```python
from build123d import *

# Parameters (mm, degrees)
BOSS_EXTRUDE1_DEPTH      = 1.5
BOSS_EXTRUDE1_DEPTH_BACK = 1.5
BOSS_EXTRUDE2_DEPTH      = 1.5
BOSS_EXTRUDE2_DEPTH_BACK = 1.5
SKETCH4_W                = 11.052180397
SKETCH4_H                = 1.65
SKETCH5_R                = 1.4
BOSS_EXTRUDE20_DEPTH     = 3.5
SKETCH6_R                = 26
SKETCH6_R_2              = 25
CUT_EXTRUDE1_DEPTH       = 1.65


with BuildPart() as part:
    # Sketch1 → Revolve1 (revolve)
    with BuildSketch(Plane.XY, mode=Mode.PRIVATE) as revolve1_sk:
        with BuildLine():
            Line((-20.885, 0), (-20.885, 11.793939121))
            ThreePointArc((-20.885, 11.793939121), (-12.091372858, 20.714220415), (0, 23.985))
            Line((0, 23.985), (0, 25.485))
            ThreePointArc((0, 25.485), (-18.020616319, 18.020616319), (-25.485, 0))
            Line((-25.485, 0), (-24.285, 0))
            Line((-24.285, 0), (-24.285, 0.5))
            Line((-24.285, 0.5), (-22.085, 0.5))
            Line((-22.085, 0.5), (-22.085, 0))
            Line((-22.085, 0), (-20.885, 0))
        make_face()
    revolve(revolve1_sk.sketch.rotate(Axis((0, 0, 0), (0, 1, 0)), 270), axis=Axis((0, 0, 0), (0, 1, 0)))



with BuildPart() as body_2:
    # Sketch2 → Boss-Extrude1 (new, two sides)
    with BuildSketch(Plane.XY) as boss_extrude1_sk:
        with BuildLine():
            Line((-24.9, 0), (-35, 0))
            ThreePointArc((-35, 0), (0, 35), (35, 0))
            Line((35, 0), (24.9, 0))
            ThreePointArc((24.9, 0), (0, 24.9), (-24.9, 0))
        make_face()
    extrude(amount=BOSS_EXTRUDE1_DEPTH)
    extrude(boss_extrude1_sk.sketch, amount=-BOSS_EXTRUDE1_DEPTH_BACK)

    # Sketch3 → Boss-Extrude2 (add, two sides)
    with BuildSketch(Plane(origin=(0, 0, 0), x_dir=(0, 0, -1), z_dir=(1, 0, 0))) as boss_extrude2_sk:
        with BuildLine():
            Line((35, 0), (24.9, 0))
            ThreePointArc((24.9, 0), (0, 24.9), (-24.9, 0))
            Line((-24.9, 0), (-35, 0))
            ThreePointArc((-35, 0), (0, 35), (35, 0))
        make_face()
    extrude(amount=BOSS_EXTRUDE2_DEPTH)
    extrude(boss_extrude2_sk.sketch, amount=-BOSS_EXTRUDE2_DEPTH_BACK)

    # Sketch4 → Cut-Revolve2 (revolve, cut)
    with BuildSketch(Plane.XY):
        with Locations((-30.371361379, 0.825)):
            Rectangle(SKETCH4_W, SKETCH4_H)
    revolve(axis=Axis((0, 0, 0), (0, 1, 0)), mode=Mode.SUBTRACT)


with BuildPart() as part_1:
    add(part.part)

    add(body_2.part)  # Boss-Extrude20 merges body 2
    # Sketch5 → Boss-Extrude20 (add)
    with BuildSketch(Plane.XZ.offset(-1.65)):
        with BuildLine():
            Line((-32.23863084, -1.5), (-24.23863084, -1.5))
            ThreePointArc((-24.23863084, -1.5), (-23.660511509, -5.471875377), (-22.4360777, -9.294280094))
            ThreePointArc((-22.4360777, -9.294280094), (-27.026694315, -8.998446643), (-30.695451754, -6.223289498))
            ThreePointArc((-30.695451754, -6.223289498), (-31.843056108, -3.984495189), (-32.23863084, -1.5))
        make_face()
        with Locations(Location((-28.212839525, -4.2, 0), (0, 0, 270))):
            Circle(SKETCH5_R, mode=Mode.SUBTRACT)
        with BuildLine():
            Line((24.23863084, 1.5), (32.23863084, 1.5))
            ThreePointArc((32.23863084, 1.5), (31.843056108, 3.984495189), (30.695451754, 6.223289498))
            ThreePointArc((30.695451754, 6.223289498), (27.026694315, 8.998446643), (22.4360777, 9.294280094))
            ThreePointArc((22.4360777, 9.294280094), (23.660511509, 5.471875377), (24.23863084, 1.5))
        make_face()
        with Locations(Location((28.212839525, 4.2, 0), (0, 0, 270))):
            Circle(SKETCH5_R, mode=Mode.SUBTRACT)
        with BuildLine():
            Line((-1.5, 32.23863084), (-1.5, 24.23863084))
            ThreePointArc((-1.5, 24.23863084), (-5.471875377, 23.660511509), (-9.294280094, 22.4360777))
            ThreePointArc((-9.294280094, 22.4360777), (-8.998446643, 27.026694315), (-6.223289498, 30.695451754))
            ThreePointArc((-6.223289498, 30.695451754), (-3.984495189, 31.843056108), (-1.5, 32.23863084))
        make_face()
        with Locations(Location((-4.2, 28.212839525, 0), (0, 0, 270))):
            Circle(SKETCH5_R, mode=Mode.SUBTRACT)
        with BuildLine():
            Line((1.5, -32.23863084), (1.5, -24.23863084))
            ThreePointArc((1.5, -24.23863084), (5.471875377, -23.660511509), (9.294280094, -22.4360777))
            ThreePointArc((9.294280094, -22.4360777), (8.998446643, -27.026694315), (6.223289498, -30.695451754))
            ThreePointArc((6.223289498, -30.695451754), (3.984495189, -31.843056108), (1.5, -32.23863084))
        make_face()
        with Locations(Location((4.2, -28.212839525, 0), (0, 0, 270))):
            Circle(SKETCH5_R, mode=Mode.SUBTRACT)
    extrude(amount=-BOSS_EXTRUDE20_DEPTH)

    # Sketch6 → Cut-Extrude1 (cut)
    with BuildSketch(Plane.XZ):
        Circle(SKETCH6_R)
        with Locations(Location((0, 0, 0), (0, 0, 270))):
            Circle(SKETCH6_R_2, mode=Mode.SUBTRACT)
    extrude(amount=-CUT_EXTRUDE1_DEPTH, mode=Mode.SUBTRACT)

    # SurfaceCut1
    split(bisect_by=Plane(origin=(0, 0, 0), x_dir=(0, 0, -1), z_dir=(1, 0, 0)), keep=Keep.TOP)


solid = part_1.part
```
Verification items for the finished model (mm, model axes). A direction names the side the tool comes from. Give positions to 0.01 mm unless a question says otherwise; leave off trailing zeros. Write each loop counter-clockwise with the first axis right and the second up, starting at its lowest first coordinate (ties: lowest second). Pieces come first, ordered by that corner, then holes. Notation, with made-up numbers: M 26,-35 L 32,-35 A5 ccw 32,-28 Z; hole C 45,27.5 d4. An arc over 180 degrees is marked long. One line per question, with ' | ' between items.
1) Mould release check, pull along X, two halves, no side actions. Record for faces 5 (the cylindrical face through (24.28, 0.25, 0.53)), 6 (the flat face through (28, 5.15, 6)), 7 (the flat face through (0, 26, 0)): released by +X, released by -X, zero draft, split by the parting line, or undercut.
Result:
face 5: undercut | face 6: zero draft | face 7: released by -X
2) Section check A-A on z = 4.2. Enter the section's corners in (x, y).
Result:
outline: M 0,23.61 A23.61 cw 20.46,11.79 L 20.46,0 L 21.68,0 L 21.68,0.5 L 23.92,0.5 L 23.92,0 L 24.64,0 L 24.64,1.65 L 26.81,1.65 L 26.81,5.15 L 24.6,5.15 A25.14 ccw 1.5,25.09 L 1.5,34.75 L 0,34.75 Z; M 29.61,1.65 L 31.77,1.65 L 31.77,5.15 L 29.61,5.15 Z
3) Gauge pin test, flat ends, axial feed: pin 1 Ø3 at (x, z) = (28.21, 4.2) entering from +Y; pin 2 Ø8 at (y, z) = (22.5, 16.5) entering from -X; pin 3 Ø1 at (y, z) = (5.5, -15.5) entering from +X; pin 4 Ø6 at (x, y) = (15, 20) entering from -Z. Record the tip position at first contact, or that the pin passes through.
Result:
pin 1: stops at y = 5.15 | pin 2: stops at x = 0 | pin 3: stops at x = 19.88 | pin 4: stops at z = -12.86
4) Section check C-C on y = 20. Enter the section's corners in (x, z), plus the area to 3 significant figures.
Result:
outline: M 0,-28.72 L 1.5,-28.72 L 1.5,-15.72 A15.8 ccw 15.72,-1.5 L 28.72,-1.5 L 28.72,1.5 L 15.72,1.5 A15.8 ccw 1.5,15.72 L 1.5,28.72 L 0,28.72 L 0,13.24 A13.24 cw 0,-13.24 Z | area: 194 mm2
5) Section check B-B on x = 4.2. Enter the section's corners in (y, z).
Result:
outline: M 0,-24.64 L 1.65,-24.64 L 1.65,-26.81 L 5.15,-26.81 L 5.15,-24.6 A25.14 ccw 25.09,-1.5 L 34.75,-1.5 L 34.75,1.5 L 25.09,1.5 A25.14 ccw 1.65,25.08 L 1.65,24.64 L 0,24.64 L 0,23.92 L 0.5,23.92 L 0.5,21.68 L 0,21.68 L 0,20.46 L 11.79,20.46 A23.61 cw 11.79,-20.46 L 0,-20.46 L 0,-21.68 L 0.5,-21.68 L 0.5,-23.92 L 0,-23.92 Z; M 1.65,-31.77 L 5.15,-31.77 L 5.15,-29.61 L 1.65,-29.61 Z
6) Thickness scan on line 1 along Z through (x, y) = (24, 23.5); line 2 along Z through (x, y) = (4, 4); line 3 along Z through (x, y) = (16, 14). Record the ranges inside material, lowest first. Write a range as [from, to].
Result:
line 1: z = [-1.5, 1.5] | line 2: z = [-31.84, -29.6], [-26.83, -20.5], [20.5, 24.85] | line 3: z = [-14.05, -11.1], [11.1, 14.05]
7) Set-up check for faces 1 (the cylindrical face through (24.994, 0.813, -0.55)), 2 (the cylindrical face through (22.08, 0.25, 0.49)), 3 (the cylindrical face through (20.88, 5.98, 0.46)), 4 (the flat face through (18, 19, -1.5)): record each of +Z, -Z, +X, -X, +Y, -Y from which the full face is reachable in a straight line by a thin tool's end or side.
Result:
face 1: +X, -Y | face 2: -Y | face 3: -X, -Y | face 4: -Z, +X, +Y
8) Section check D-D on x = 16. Enter the section's corners in (y, z), plus the area to 3 significant figures.
Result:
outline: M 0,-19.21 L 1.65,-19.21 L 1.65,-19.77 A19.84 ccw 19.78,-1.5 L 31.13,-1.5 L 31.13,1.5 L 19.78,1.5 A19.84 ccw 1.65,19.77 L 1.65,19.21 L 0,19.21 L 0,18.27 L 0.5,18.27 L 0.5,15.22 L 0,15.22 L 0,13.42 L 11.79,13.42 A17.87 cw 11.79,-13.42 L 0,-13.42 L 0,-15.22 L 0.5,-15.22 L 0.5,-18.27 L 0,-18.27 Z | area: 217 mm2
